Autodesk Inventor part; units mm, degrees
ref_plane "XZ Plane" through (0, 0, 0) normal (0, 1, 0) x (-1, 0, 0)
ref_plane "XY Plane" through (0, 0, 0) normal (0, 0, 1) x (1, 0, 0)
sketch "Sketch1" plane through (0, 0, 0) normal (0, 1, 0) x (-1, 0, 0)
  circle A0 centre (0, 0) radius 1.1
  circle A1 centre (0, 0) radius 2.575
  dimension "d0" = 2.2
  dimension "d1" = 5.15
extrude "Extrusion1" add sketch "Sketch1" along normal blind 18
sketch "Sketch2" plane through (0, 0, 0) normal (0, 0, 1) x (1, 0, 0)
  line L0 (2.575, 18) -> (-2.575, 18)
  line L1 (2.575, 0) -> (-2.575, 0)
  line L2 (-2.575, 0) -> (-2.575, 18)
  line L3 (-2.575, 16) -> (2.5173, 16)
  line L4 (2.575, 18) -> (-2.575, 18)
  line L5 (0, 18) -> (0, 0)
  circle A0 centre (0, 13.9) radius 2.1
  dimension "d4" = 2
  dimension "d5" = 4.2
extrude "Extrusion2" cut sketch "Sketch2" along normal blind 12 contours A0 L5 | L5 A0
sketch "Sketch3" plane through (0, 0, 0) normal (1, 0, 0) x (0, 1, 0)
  line L0 (18, -2.575) -> (18, 2.575)
  line L1 (0, -2.575) -> (0, 2.575)
  line L2 (0, 2.575) -> (18, 2.575)
  line L3 (16, 2.575) -> (16, -2.525)
  line L4 (18, 1.1) -> (18, -1.1)
  line L5 (18, 0) -> (0, 0)
  circle A0 centre (13.9, 0) radius 2.1
  point P0 (13.9, 1.4902)
  dimension "d8" = 2
  dimension "d9" = 4.2
extrude "Extrusion3" cut sketch "Sketch3" along normal up to next contours A0 L5 | L5 A0
properties part number "motor_shaft_adapter"
Input: part model. Units: mm. Frame: model coordinates. A direction names the side the tool comes from. Give positions to 0.01 mm unless a question says otherwise; leave off trailing zeros. Loops run counter-clockwise (first coordinate to the right, second up) from the corner with the lowest first, then second, coordinate; pieces in that order, holes last. Notation, with made-up numbers: (19, 41) -> (77, 41) arc R22 cw to (77, 71) -> close; hole circle Ø8 at (-34, 10.25). An arc over 180 degrees is marked (long way). Use a Markdown table: item, result.
Q1. Section query D-D, the plane x = -1.7. Return the cut outline in (y, z), plus the area to 3 significant figures.
Entries:
| item | result |
|---|---|
| outline | (0, -1.93) -> (18, -1.93) -> (18, 1.93) -> (15.13, 1.93) -> (15.13, 0) -> (12.67, 0) -> (12.67, 1.93) -> (0, 1.93) -> close |
| area | 64.9 mm² |
Q2. Pull-direction query (X, two-part tool) for faces 3 (the cylindrical face through (-1.05, 6.87, -0.33)), 4 (the flat face through (0, 13.9, -1.5)), 5 (the cylindrical face through (-2.1, 13.82, 0.98)), 6 (the flat face through (-1.5, 13.9, 0)); classes: pulls with the +X half, pulls with the -X half, needs draft (parallel to the pull), parting line crosses it, or undercut.
Entries:
| item | result |
|---|---|
| face 3 | undercut |
| face 4 | pulls with the +X half |
| face 5 | undercut |
| face 6 | needs draft |
Q3. Access query for faces 1 (the cylindrical face through (0.98, 13.98, -2.1)), 2 (the flat face through (-1, 18, -1)). Directions: +Z, -Z, +X, -X, +Y, -Y. A direction counts if a zero-diameter tool reaches every point of the face in a straight line with its end or side. Return the directions, or none.
Entries:
| item | result |
|---|---|
| face 1 | +X |
| face 2 | +Z, -Z, +X, -X, +Y |
Q4. Ray query, probe 1 along X at (y, z) = (8, 0) (3 decimals); probe 2 along Y at (x, z) = (1.3, 0.1); probe 3 along Y at (x, z) = (1.05, -1.15). Return the intervals inside material, ascending. Write a range as from..to.
Entries:
| item | result |
|---|---|
| probe 1 | x = -2.575..-1.1, 1.1..2.575 |
| probe 2 | y = 0..11.8, 16..18 |
| probe 3 | y = 0..12.14, 15.66..18 |
Q5. Section query A-A, the plane z = -0.35. Return the cut outline in (x, y).
Entries:
| item | result |
|---|---|
| outline | (-2.55, 0) -> (-1.04, 0) -> (-1.04, 18) -> (-2.55, 18) -> close; (1.04, 0) -> (2.55, 0) -> (2.55, 11.83) -> (1.04, 11.83) -> close; (1.04, 15.97) -> (2.55, 15.97) -> (2.55, 18) -> (1.04, 18) -> close |
Q6. Section query B-B, the plane x = 0.2. Return the cut outline in (y, z), plus the area to 3 significant figures.
Entries:
| item | result |
|---|---|
| outline | (0, -2.57) -> (18, -2.57) -> (18, -1.08) -> (15.7, -1.08) arc R2.1 cw to (12.1, -1.08) -> (0, -1.08) -> close; (0, 1.08) -> (11.81, 1.08) -> (11.81, 2.57) -> (0, 2.57) -> close; (15.99, 1.08) -> (18, 1.08) -> (18, 2.57) -> (15.99, 2.57) -> close |
| area | 44.7 mm² |
Q7. Section query C-C, the plane y = 6.5. Return the cut outline in (x, z) (3 decimals), plus the area to 3 significant figures.
Entries:
| item | result |
|---|---|
| outline | circle Ø5.15 at (0, 0); hole circle Ø2.2 at (0, 0) |
| area | 17.0 mm² |
Q8. First-contact query: P1, Ø1, axis at x = -1, y = 12, coming from the +Z side; P2, Ø1.1, axis at y = 13.5, z = -2, coming from the +X side; P3, Ø1.5, axis at x = -2, y = 13, coming from the -Z side. Flat tips, straight axial feed; report the tip coordinate or a pass-through.
Entries:
| item | result |
|---|---|
| P1 | stops at z = 2.52 |
| P2 | stops at x = 1.76 |
| P3 | stops at z = -2.25 |
